Part model, mm, in its own coordinate system. Face numbers are marked on the shaded views. A direction names the side the tool comes from. Round coordinates to 2 decimals unless told otherwise and drop trailing zeros. Loops run counter-clockwise (first coordinate to the right, second up) from the corner with the lowest first, then second, coordinate; pieces in that order, holes last. Notation, with made-up numbers: (-27, 22.5) - (-20, 22.5) arc R26 ccw to (-20, 49.5) - close; hole circle Ø3 at (-6.75, 79). An arc over 180 degrees is marked (long way). Put each result on its own line as item: value.
from build123d import *

# Parameters (mm, degrees)
F0_W      = 39
F0_H      = 51
F0_R      = 1.5
F1_DEPTH  = 1.6
F2_W      = 15
F2_H      = 18.5
F3_DEPTH  = 15
F4_W      = 31
F4_H      = 8
F5_DEPTH  = 10
F6_SIZE   = 2
F7_R      = 1.5
F8_DEPTH  = 3
F9_W      = 4
F9_H      = 6
F10_DEPTH = 4
F11_W     = 7
F11_H     = 1.406925
F11_W_2   = 10
F12_DEPTH = 2.5
F13_W     = 0.5
F13_H     = 0.5
F14_DEPTH = 6


with BuildPart() as f1:
    # F0 (on Top) → F1 (new body)
    with BuildSketch(Plane.XY):
        Rectangle(F0_W, F0_H)
        with Locations((-16.9, -22.9)):
            Circle(F0_R, mode=Mode.SUBTRACT)
        with Locations((16.9, -22.9)):
            Circle(F0_R, mode=Mode.SUBTRACT)
        with Locations((-16.9, 22.9)):
            Circle(F0_R, mode=Mode.SUBTRACT)
        with Locations((16.9, 22.9)):
            Circle(F0_R, mode=Mode.SUBTRACT)
    extrude(amount=F1_DEPTH)

    # F2 (on face) → F3 (join)
    with BuildSketch(Plane.XY.offset(1.6)):
        with Locations((-8, 3.75)):
            Rectangle(F2_W, F2_H)
        with Locations((8, 3.75)):
            Rectangle(F2_W, F2_H)
    extrude(amount=F3_DEPTH)

    # F4 (on face) → F5 (join)
    with BuildSketch(Plane.XY.offset(1.6)):
        with Locations((0, 17.5)):
            Rectangle(F4_W, F4_H)
    extrude(amount=F5_DEPTH)

    # F6
    f6_edges = [f1.edges().sort_by_distance(p)[0] for p in [
        (0, 13.5, 11.6),
    ]]
    chamfer(f6_edges, length=F6_SIZE)

    # F7 (on face) → F8 (cut)
    with BuildSketch(Plane.XY.offset(11.6)):
        with Locations((-13.25, 18.5)):
            Circle(F7_R)
        with Locations((-8.25, 18.5)):
            Circle(F7_R)
        with Locations((-3.25, 18.5)):
            Circle(F7_R)
        with Locations((3.386981, 18.5)):
            Circle(F7_R)
        with Locations((8.386981, 18.5)):
            Circle(F7_R)
        with Locations((13.386981, 18.5)):
            Circle(F7_R)
    extrude(amount=-F8_DEPTH, mode=Mode.SUBTRACT)

    # F9 (on face) → F10 (join)
    with BuildSketch(Plane.XY.offset(1.6)):
        with Locations((-3, -13.5)):
            Rectangle(F9_W, F9_H)
        with Locations((3, -13.5)):
            Rectangle(F9_W, F9_H)
    extrude(amount=F10_DEPTH)

    # F11 (on face) → F12 (join)
    with BuildSketch(Plane.XY.offset(1.6)):
        with Locations((-4.5, -22.796537)):
            Rectangle(F11_W, F11_H)
        with Locations((6, -22.796537)):
            Rectangle(F11_W_2, F11_H)
    extrude(amount=F12_DEPTH)

    # F13 (on face) → F14 (join)
    with BuildSketch(Plane.XY.offset(4.1)):
        with Locations((-7, -22.75)):
            Rectangle(F13_W, F13_H)
        with Locations((-4.46, -22.75)):
            Rectangle(F13_W, F13_H)
        with Locations((-1.92, -22.75)):
            Rectangle(F13_W, F13_H)
        with Locations((2.38, -22.75)):
            Rectangle(F13_W, F13_H)
        with Locations((4.92, -22.75)):
            Rectangle(F13_W, F13_H)
        with Locations((7.46, -22.75)):
            Rectangle(F13_W, F13_H)
        with Locations((10, -22.75)):
            Rectangle(F13_W, F13_H)
    extrude(amount=F14_DEPTH)


solid = f1.part
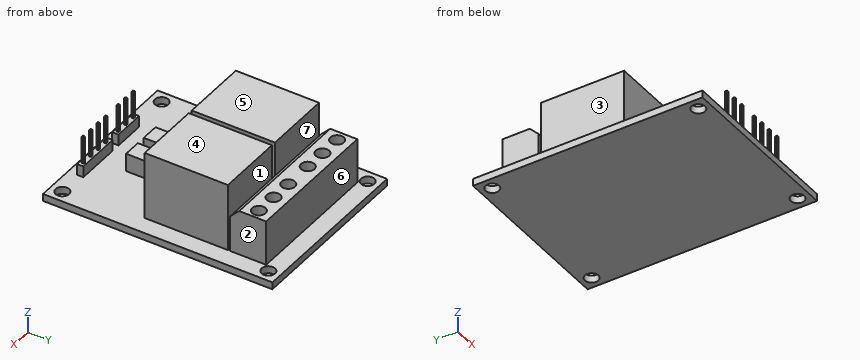
1. Band-saw the part on B-B (y = 22.9). List the corners of the cut face in (x, z), plus the area to 3 significant figures.
A:
outline: (-19.5, 0) - (-18.4, 0) - (-18.4, 1.6) - (-19.5, 1.6) - close; (-15.4, 0) - (15.4, 0) - (15.4, 1.6) - (-15.4, 1.6) - close; (18.4, 0) - (19.5, 0) - (19.5, 1.6) - (18.4, 1.6) - close
area: 52.8 mm²
2. Tool access for the marked faces 1, 2, 3 and 4: list every direction of +Z, -Z, +X, -X, +Y, -Y with a clear straight run to the whole face (end or side of a thin tool).
A:
face 1: +Z, +X, -X
face 2: +Z, +X, +Y, -Y
face 3: +Z, -X, +Y, -Y
face 4: +Z, +X, -X, +Y, -Y
3. Pin check, flat tips, straight feed: P1, Ø1.2, axis at y = -14, z = 3, coming from the +X side; P2, Ø2, axis at x = -7, z = 11.5, coming from the -Y side; P3, Ø2.5, axis at x = -13.25, y = 18.5, coming from the +Z side. Stop position of each tip, or through.
A:
P1: stops at x = 5
P2: stops at y = -5.5
P3: stops at z = 8.6
4. Two-plate mould, pull along Y, no slides. Class the marked faces 5, 6 and 7: pulls with the +Y half, pulls with the -Y half, needs draft (parallel to the pull), parting line crosses it, or undercut.
A:
face 5: needs draft
face 6: pulls with the +Y half
face 7: undercut
5. Probe line 1 along Y through (x, z) = (6, 3); line 2 along Y through (x, z) = (16.9, 1); line 3 along Y through (x, z) = (4.5, 6.75). List the from-to ranges inside material, lowest first. Write a range as [from, to].
A:
line 1: y = [-23.5, -22.09], [-5.5, 13], [13.5, 21.5]
line 2: y = [-25.5, -24.4], [-21.4, 21.4], [24.4, 25.5]
line 3: y = [-5.5, 13], [13.5, 21.5]
6. Band-saw the part on C-C (z = 13.5). List the corners of the cut face in (x, y).
A:
outline: (-15.5, -5.5) - (-0.5, -5.5) - (-0.5, 13) - (-15.5, 13) - close; (0.5, -5.5) - (15.5, -5.5) - (15.5, 13) - (0.5, 13) - close
7. Band-saw the part on D-D (z = 3.5). List the corners of the cut face in (x, y).
A:
outline: (-15.5, -5.5) - (-0.5, -5.5) - (-0.5, 13) - (-15.5, 13) - close; (-15.5, 13.5) - (15.5, 13.5) - (15.5, 21.5) - (-15.5, 21.5) - close; (-8, -23.5) - (-1, -23.5) - (-1, -22.09) - (-8, -22.09) - close; (-5, -16.5) - (-1, -16.5) - (-1, -10.5) - (-5, -10.5) - close; (0.5, -5.5) - (15.5, -5.5) - (15.5, 13) - (0.5, 13) - close; (1, -23.5) - (11, -23.5) - (11, -22.09) - (1, -22.09) - close; (1, -16.5) - (5, -16.5) - (5, -10.5) - (1, -10.5) - close
8. Band-saw the part on A-A (x = 16.9). List the corners of the cut face in (y, z).
A:
outline: (-25.5, 0) - (-24.4, 0) - (-24.4, 1.6) - (-25.5, 1.6) - close; (-21.4, 0) - (21.4, 0) - (21.4, 1.6) - (-21.4, 1.6) - close; (24.4, 0) - (25.5, 0) - (25.5, 1.6) - (24.4, 1.6) - close
